Verification items for the finished model (mm, model axes). A direction names the side the tool comes from. Give positions to 0.01 mm unless a question says otherwise; leave off trailing zeros. Loops run counter-clockwise (first coordinate to the right, second up) from the corner with the lowest first, then second, coordinate; pieces in that order, holes last. Notation, with made-up numbers: M 38,55.5 L 97,55.5 A12 cw 97,69.5 Z; hole C 9,45 d9. An arc over 180 degrees is marked long. Write each question's results on one line, items separated by ' | '. Start each with the question number.
Autodesk Inventor part; units mm, degrees
ref_plane "YZ Plane" through (0, 0, 0) normal (1, 0, 0) x (0, 1, 0)
ref_plane "XZ Plane" through (0, 0, 0) normal (0, 1, 0) x (-1, 0, 0)
ref_plane "XY Plane" through (0, 0, 0) normal (0, 0, 1) x (1, 0, 0)
sketch "Skizze1" plane through (0, 0, 0) normal (0, 0, 1) x (1, 0, 0)
  line L0 (55, -68) -> (-55, -68)
  line L1 (-55, -68) -> (-55, 68)
  line L2 (-55, 68) -> (55, 68)
  line L3 (55, 68) -> (55, -68)
  line L4 (55, -68) -> (-55, 68) construction
  line L5 (-55, -68) -> (55, 68) construction
  point P0 (0, 0)
  dimension "d0" = 110
  dimension "d1" = 136
extrude "Extrusion1" add sketch "Skizze1" along normal blind 2
sketch "Skizze2" plane through (0, 0, 0) normal (0, 0, 1) x (1, 0, 0)
  line L0 (-22.5, 23) -> (22.5, 23)
  line L1 (22.5, 23) -> (22.5, 60)
  line L2 (22.5, 60) -> (-22.5, 60)
  line L3 (-22.5, 60) -> (-22.5, 23)
  line L4 (-22.5, 23) -> (22.5, 60) construction
  line L5 (22.5, 23) -> (-22.5, 60) construction
  line L6 (55, 68) -> (-55, 68)
  line L7 (-3.5, 13) -> (3.5, 13)
  line L8 (3.5, 13) -> (3.5, 23)
  line L9 (3.5, 23) -> (-3.5, 23)
  line L10 (-3.5, 23) -> (-3.5, 13)
  line L11 (-3.5, 13) -> (3.5, 23) construction
  line L12 (3.5, 13) -> (-3.5, 23) construction
  point P0 (0, 0)
  point P1 (0, 41.5)
  point P2 (0, 18)
  dimension "d4" = 45
  dimension "d5" = 37
  dimension "d6" = 8
  dimension "d7" = 7
  dimension "d8" = 10
extrude "Extrusion2" add sketch "Skizze2" against normal blind 8
equation "\"d0\" = SolarPanelWidth"
equation "\"d1\" = SolarPanelHeight"
equation "\"d2\" = SolarPanelThickness"
equation "\"d4\" = SolarPanelConnectorWidth"
equation "\"d5\" = SolarPanelConnectorHeight"
equation "\"d9\" = SolarPanelConnectorDepth"
properties part number "SolarPanel"
1. Thickness scan on probe 1 along Z at (x, y) = (23, 54); probe 2 along Y at (x, z) = (-22, -6). Record the ranges inside material, lowest first.
2. Section check C-C, the plane y = -1. Record the boundary of the cut face in (x, z).
3. Set-up check for faces 1 (the face through (13, 23, -4)), 2 (the face through (22.5, 41, -4)), 3 (the face through (-3.5, 18, -4)): record each of +Z, -Z, +X, -X, +Y, -Y from which the full face is reachable in a straight line by a thin tool's end or side.
4. Section check A-A, the plane z = -2. Record the boundary of the cut face in (x, y).
5. Section check B-B, the plane x = 16. Record the boundary of the cut face in (y, z), plus the area to 3 significant figures.
6. Depth check by flat-ended pin: pin 1 Ø3.5 at (x, z) = (-0.5, -4.5) entering from -Y; pin 2 Ø10 at (x, y) = (1, 6) entering from -Z; pin 3 Ø4 at (y, z) = (20.5, -4) entering from -X. Enter the tip coordinate at first touch or a pass-through.
7. Section check D-D, the plane x = 40.5. Record the boundary of the cut face in (y, z), plus the area to 3 significant figures.
Filled sheet:
1) probe 1: 0 to 2 | probe 2: 23 to 60
2) outline: M -55,0 L 55,0 L 55,2 L -55,2 Z
3) face 1: -Z, +X, -Y | face 2: -Z, +X, +Y, -Y | face 3: -Z, -X, -Y
4) outline: M -22.5,23 L -3.5,23 L -3.5,13 L 3.5,13 L 3.5,23 L 22.5,23 L 22.5,60 L -22.5,60 Z
5) outline: M -68,0 L 23,0 L 23,-8 L 60,-8 L 60,0 L 68,0 L 68,2 L -68,2 Z | area: 568 mm2
6) pin 1: y = 13 | pin 2: z = 0 | pin 3: x = -3.5
7) outline: M -68,0 L 68,0 L 68,2 L -68,2 Z | area: 272 mm2
